The listing builds one solid part. Answer for the finished solid, in the listing's coordinates (mm). A direction names the side the tool comes from. Give positions to 0.01 mm unless a question says otherwise; leave off trailing zeros. Loops run counter-clockwise (first coordinate to the right, second up) from the corner with the lowest first, then second, coordinate; pieces in that order, holes last. Notation, with made-up numbers: (80.5, 34) - (116.5, 34) arc R16 cw to (116.5, 41) - close; hole circle Ø9 at (36, -16.5). An arc over 180 degrees is marked (long way). Answer as CSV lines item,"result". Start each with the question number.
1) For faces 4 (the face through (-5.03, 35.91, 1.58)), 5 (the face through (-3, 35, 0)), determine the directions among +Z, -Z, +X, -X, +Y, -Y from which every point of the face is accessible in a straight line to the end or side of a thin tool.
2) Flat-ended cylindrical pins translate along their axes: pin 1 (4 mm diameter, centred on y = 29, z = 2, fed in from -X); pin 2 (2 mm diameter, centred on x = -2.5, y = 40.5, fed in from +Z); pin 3 (4 mm diameter, centred on y = 40, z = 2, fed in from +X). Find the tip coordinate at first contact, or state that the pin passes through.
3) Find the intervals of material crossed by line 1 along Z through (x, y) = (0, 26.2); line 2 along Z through (x, y) = (1.5, 26); line 3 along X through (y, z) = (28.75, 1.75), in increasing order.
4) A cutting plane is placed at A-A (y = 28.25). Determine the outline of the cut face in (x, z), and give its area (3 significant figures).
5) A cutting plane is placed at B-B (y = 35.5). Determine the outline of the cut face in (x, z), and give its area (3 significant figures).
6) For a pull along X with two mould halves and no side action, classify faces 1 (the face through (0.845, 29.019, -3.806)), 2 (the face through (0, 33.503, -5)), 3 (the face through (3, 27.9, 1)) as pulls with the +X half, pulls with the -X half, needs draft (parallel to the pull), parting line crosses it, or undercut.
```python
from build123d import *

# Parameters (mm, degrees)
M7X1_0_TAPPED_HOLE1_D     = 6
M7X1_0_TAPPED_HOLE1_DEPTH = 16.002
M7X1_0_TAPPED_HOLE1_TIP   = 1.802581857
SKETCH4_R                 = 3.5
CUT_EXTRUDE1_DEPTH        = 2.5
FILLET1_R                 = 0.762


with BuildPart() as part:
    # Sketch1 → Revolve1 (revolve)
    with BuildSketch(Plane.XY):
        with BuildLine():
            Line((-5.2705, 38.3921), (-5.2705, 33.5026))
            Line((-5.2705, 33.5026), (-3.899, 33.5026))
            Line((-3.899, 33.5026), (-3.899, 25.4))
            Line((-3.899, 25.4), (0, 25.4))
            Line((0, 25.4), (0, 43.6626))
            ThreePointArc((0, 43.6626), (-3.72680629, 42.11890629), (-5.2705, 38.3921))
        make_face()
    revolve(axis=Axis((0, 25.4, 0), (0, 1, 0)))

    # M7x1.0 Tapped Hole1
    with Locations(Plane(origin=(0, 25.4, 0), x_dir=(-1, 0, 0), z_dir=(0, -1, 0))):
        with Locations((0, 0)):
            Hole(M7X1_0_TAPPED_HOLE1_D / 2, depth=M7X1_0_TAPPED_HOLE1_DEPTH)
            with Locations((0, 0, -(M7X1_0_TAPPED_HOLE1_DEPTH + M7X1_0_TAPPED_HOLE1_TIP / 2))):  # 118° drill point
                Cone(0, M7X1_0_TAPPED_HOLE1_D / 2, M7X1_0_TAPPED_HOLE1_TIP, mode=Mode.SUBTRACT)

    # Sketch4 → Cut-Extrude1 (cut)
    with BuildSketch(Plane.XZ.offset(-25.4)):
        Circle(SKETCH4_R)
    extrude(amount=-CUT_EXTRUDE1_DEPTH, mode=Mode.SUBTRACT)

    # Fillet1
    fillet1_edges = [part.edges().sort_by_distance(p)[0] for p in [
        (3.899, 33.5026, 0),
    ]]
    fillet(fillet1_edges, radius=FILLET1_R)


solid = part.part
```
Ans:
1,face 4,"+Y, -Y"
1,face 5,"-Y"
2,pin 1,"x = -3.9"
2,pin 2,"z = 4.76"
2,pin 3,"x = 5.24"
3,line 1,"-3.9 to -3.5, 3.5 to 3.9"
3,line 2,"-3.6 to -3.16, 3.16 to 3.6"
3,line 3,"-3.48 to -2.44, 2.44 to 3.48"
4,outline,"circle Ø7.8 at (0, 0); hole circle Ø6 at (0, 0)"
4,area,"19.5 mm2"
5,outline,"circle Ø10.54 at (0, 0); hole circle Ø6 at (0, 0)"
5,area,"59.0 mm2"
6,face 1,"parting line crosses it"
6,face 2,"needs draft"
6,face 3,"undercut"
